CAD build for the part. Positions are in the model's coordinates, mm. Round coordinates to 2 decimals unless told otherwise and drop trailing zeros. Loops run counter-clockwise (first coordinate to the right, second up) from the corner with the lowest first, then second, coordinate; pieces in that order, holes last.
from build123d import *

# Parameters (mm, degrees)
SKETCH_1_R      = 4.8
EXTRUDE_1_DEPTH = 5
CHAMFER_1_SIZE  = 0.3
SKETCH_2_R      = 0.3
EXTRUDE_2_DEPTH = 5.1


with BuildPart() as part:
    # 草图1 → 凸台-拉伸1 (new body)
    with BuildSketch(Plane(origin=(0, 0, 0), x_dir=(1, 0, 0), z_dir=(0, 1, 0))):
        Circle(SKETCH_1_R)
    extrude(amount=EXTRUDE_1_DEPTH)

    # 倒角1
    chamfer_1_edges = [part.edges().sort_by_distance(p)[0] for p in [
        (-4.8, 0, 0),
        (-4.8, 5, 0),
    ]]
    chamfer(chamfer_1_edges, length=CHAMFER_1_SIZE)

    # 草图2 → 凸台-拉伸2 (add)
    with BuildSketch(Plane.XZ):
        with Locations((-2.5, 0)):
            Circle(SKETCH_2_R)
        with Locations((2.5, 0)):
            Circle(SKETCH_2_R)
    extrude(amount=EXTRUDE_2_DEPTH)


solid = part.part
Item 1: Cut at C-C (z = 0). List the corners of the cut face in (x, y), plus the area to 3 significant figures.
Verdict:
outline: (-4.8, 0.3) - (-4.5, 0) - (-2.8, 0) - (-2.8, -5.1) - (-2.2, -5.1) - (-2.2, 0) - (2.2, 0) - (2.2, -5.1) - (2.8, -5.1) - (2.8, 0) - (4.5, 0) - (4.8, 0.3) - (4.8, 4.7) - (4.5, 5) - (-4.5, 5) - (-4.8, 4.7) - close
area: 53.9 mm2
Item 2: Flat gauge pins, fed straight in: P1, Ø1.5, axis at x = -2.5, y = -2.5, coming from the +Z side; P2, Ø1.5, axis at x = -3.5, y = 3, coming from the -Z side; P3, Ø2, axis at y = 2, z = -2, coming from the -X side; P4, Ø4, axis at y = -1, z = 1, coming from the -X side. Where does each tip first touch, or does it go through?
Verdict:
P1: stops at z = 0.3
P2: stops at z = -3.93
P3: stops at x = -4.69
P4: stops at x = -4.8
Item 3: Cut at D-D (y = 1). List the corners of the cut face in (x, z), plus the area to 3 significant figures.
Verdict:
outline: circle Ø9.6 at (0, 0)
area: 72.4 mm2
Item 4: Wall check: L1, parallel to Y at x = 0.25, z = 1; L2, parallel to Z at x = 2.5, y = -3; L3, parallel to Z at x = -2.75, y = 3.5. Give the ranges that are in metal, low to high.
Verdict:
L1: y = 0 to 5
L2: z = -0.3 to 0.3
L3: z = -3.93 to 3.93
Item 5: Cut at B-B (y = -3.5). List the corners of the cut face in (x, z), plus the area to 3 significant figures.
Verdict:
outline: circle Ø0.6 at (-2.5, 0); circle Ø0.6 at (2.5, 0)
area: 0.565 mm2
Item 6: Cut at A-A (x = 0). List the corners of the cut face in (y, z).
Verdict:
outline: (0, -4.5) - (0.3, -4.8) - (4.7, -4.8) - (5, -4.5) - (5, 4.5) - (4.7, 4.8) - (0.3, 4.8) - (0, 4.5) - close
